Work out the finished part from the listing and answer in its coordinate system (mm). Face numbers are marked on the shaded views. A direction names the side the tool comes from. Coordinates: 2 decimals unless noted, no trailing zeros. Write each loop counter-clockwise with the first axis right and the second up, starting at its lowest first coordinate (ties: lowest second). Pieces come first, ordered by that corner, then holes. Notation, with made-up numbers: (-7.5, 30.25) - (50.5, 30.25) arc R14 cw to (50.5, 36.25) - close; hole circle Ø4 at (69, -21). An arc over 180 degrees is marked (long way). Use one line per item in the form item = value. Start each with the question number.
Item 1: A cutting plane is placed at D-D (z = -3.25). Write down the section's boundary in (x, y), then the cut area to 4 significant figures.
Item 2: Given pin 1 (3 mm diameter, centred on x = 96, y = -12, fed in from +Z); pin 2 (3.5 mm diameter, centred on y = -12, z = -8.5, fed in from -X); pin 3 (4 mm diameter, centred on x = 48.5, z = -17.5, fed in from -Y), each flat-ended and moving along its own axis, determine where each tip first touches the part or whether it passes through.
Item 3: A cutting plane is placed at B-B (y = -3.75). Write down the section's boundary in (x, z), then the cut area to 3 significant figures.
Item 4: A cutting plane is placed at C-C (z = -8). Write down the section's boundary in (x, y).
Item 5: A cutting plane is placed at A-A (x = 13.5). Write down the section's boundary in (y, z).
Item 6: For the marked faces 5, 6, 7, 8 and 9, determine the directions among +Z, -Z, +X, -X, +Y, -Y from which every point of the face is accessible in a straight line to the end or side of a thin tool.
Item 7: Determine the mould class of the marked faces 1, 2, 3 and 4 for opening direction X: released by +X, released by -X, zero draft, split by the parting line, or undercut.
Item 8: Consider probe 1 along X at (y, z) = (-8.25, -12); probe 2 along X at (y, z) = (-8.25, -25); probe 3 along X at (y, z) = (-4.75, -2.5). Determine where each line is inside the solid, lowest interval first.
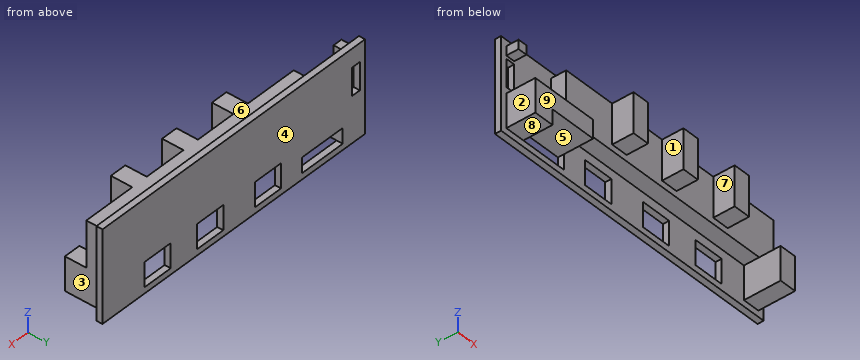
from build123d import *

# Parameters (mm, degrees)
SKETCH1_W            = 100
SKETCH1_H            = 30
SKETCH1_W_2          = 3
SKETCH1_H_2          = 9
SKETCH1_W_3          = 10
SKETCH1_H_3          = 8
SKETCH1_W_4          = 15.5
SKETCH1_H_4          = 5
BOSS_EXTRUDE3_DEPTH  = 2
SKETCH2_W            = 5.5
SKETCH2_H            = 11
BOSS_EXTRUDE4_DEPTH  = 12
BOSS_EXTRUDE5_DEPTH  = 9.5
SKETCH9_W            = 3
SKETCH9_H            = 3
BOSS_EXTRUDE17_DEPTH = 4
SKETCH12_W           = 79
SKETCH12_H           = 15
BOSS_EXTRUDE22_DEPTH = 5
SKETCH13_W           = 5.5
SKETCH13_H           = 13
BOSS_EXTRUDE23_DEPTH = 7


with BuildPart() as part:
    # Sketch1 → Boss-Extrude3 (new body)
    with BuildSketch(Plane(origin=(0, 0, 0), x_dir=(1, 0, 0), z_dir=(0, 1, 0))):
        with Locations((50, 15)):
            Rectangle(SKETCH1_W, SKETCH1_H)
        with Locations((3.5, 10.5)):
            Rectangle(SKETCH1_W_2, SKETCH1_H_2, mode=Mode.SUBTRACT)
        with Locations((79, 24)):
            Rectangle(SKETCH1_W_3, SKETCH1_H_3, mode=Mode.SUBTRACT)
        with Locations((59, 24)):
            Rectangle(SKETCH1_W_3, SKETCH1_H_3, mode=Mode.SUBTRACT)
        with Locations((37, 24)):
            Rectangle(SKETCH1_W_3, SKETCH1_H_3, mode=Mode.SUBTRACT)
        with Locations((16.25, 25.5)):
            Rectangle(SKETCH1_W_4, SKETCH1_H_4, mode=Mode.SUBTRACT)
    extrude(amount=-BOSS_EXTRUDE3_DEPTH)

    # Sketch2 → Boss-Extrude4 (add)
    with BuildSketch(Plane.XZ.offset(2)):
        with Locations((95.25, -22.5)):
            Rectangle(SKETCH2_W, SKETCH2_H)
    extrude(amount=BOSS_EXTRUDE4_DEPTH)

    # Sketch3 → Boss-Extrude5 (add)
    with BuildSketch(Plane.XZ.offset(2)):
        Polygon((24, -17), (24, -23), (8.5, -23), (8.5, -28), (2, -28), (2, -17), align=None)
    extrude(amount=BOSS_EXTRUDE5_DEPTH)

    # Sketch9 → Boss-Extrude17 (add)
    with BuildSketch(Plane.XZ.offset(2)):
        with Locations((3.5, -3.5)):
            Rectangle(SKETCH9_W, SKETCH9_H)
    extrude(amount=BOSS_EXTRUDE17_DEPTH)

    # Sketch12 → Boss-Extrude22 (add)
    with BuildSketch(Plane.XZ.offset(2)):
        with Locations((58.5, -9.5)):
            Rectangle(SKETCH12_W, SKETCH12_H)
    extrude(amount=BOSS_EXTRUDE22_DEPTH)

    # Sketch13 → Boss-Extrude23 (add)
    with BuildSketch(Plane.XZ.offset(7)):
        with Locations((39.25, -8.5)):
            Rectangle(SKETCH13_W, SKETCH13_H)
        with Locations((58.25, -8.5)):
            Rectangle(SKETCH13_W, SKETCH13_H)
        with Locations((77.75, -8.5)):
            Rectangle(SKETCH13_W, SKETCH13_H)
    extrude(amount=BOSS_EXTRUDE23_DEPTH)


solid = part.part
Answer:
q1.outline = (0, -2) - (2, -2) - (2, -6) - (5, -6) - (5, -2) - (19, -2) - (19, -7) - (36.5, -7) - (36.5, -14) - (42, -14) - (42, -7) - (55.5, -7) - (55.5, -14) - (61, -14) - (61, -7) - (75, -7) - (75, -14) - (80.5, -14) - (80.5, -7) - (98, -7) - (98, -2) - (100, -2) - (100, 0) - (0, 0) - close
q1.area = 722.5 mm²
q2.pin_1 = -17
q2.pin_2 = 36.5
q2.pin_3 = -7
q3.outline = (2, -28) - (8.5, -28) - (8.5, -23) - (24, -23) - (24, -17) - (92.5, -17) - (92.5, -28) - (98, -28) - (98, -2) - (19, -2) - (19, -17) - (2, -17) - close; (2, -5) - (5, -5) - (5, -2) - (2, -2) - close
q3.area = 1,420 mm²
q4.outline = (0, -2) - (2, -2) - (2, 0) - (0, 0) - close; (5, -2) - (19, -2) - (19, -7) - (36.5, -7) - (36.5, -14) - (42, -14) - (42, -7) - (55.5, -7) - (55.5, -14) - (61, -14) - (61, -7) - (75, -7) - (75, -14) - (80.5, -14) - (80.5, -7) - (98, -7) - (98, -2) - (100, -2) - (100, 0) - (5, 0) - close
q5.outline = (-11.5, -23) - (0, -23) - (0, 0) - (-2, 0) - (-2, -17) - (-11.5, -17) - close; (-2, -30) - (0, -30) - (0, -28) - (-2, -28) - close
q6.face_5 = +Y, -Y
q6.face_6 = +Z, +X, -X, -Y
q6.face_7 = +Z, -Z, -Y
q6.face_8 = -Z, +X, -X, -Y
q6.face_9 = +Z, -Z, -X, -Y
q7.face_1 = undercut
q7.face_2 = released by -X
q7.face_3 = released by +X
q7.face_4 = zero draft
q8.probe_1 = 36.5 to 42, 55.5 to 61, 75 to 80.5
q8.probe_2 = 2 to 8.5, 92.5 to 98
q8.probe_3 = 2 to 5, 19 to 98
